Can you work these out from the drawing? Everything is in mm from the part's minimum corner. A direction names the side the tool comes from. Round coordinates to 2 decimals unless told otherwise and drop trailing zeros. One line per item, written item: value.
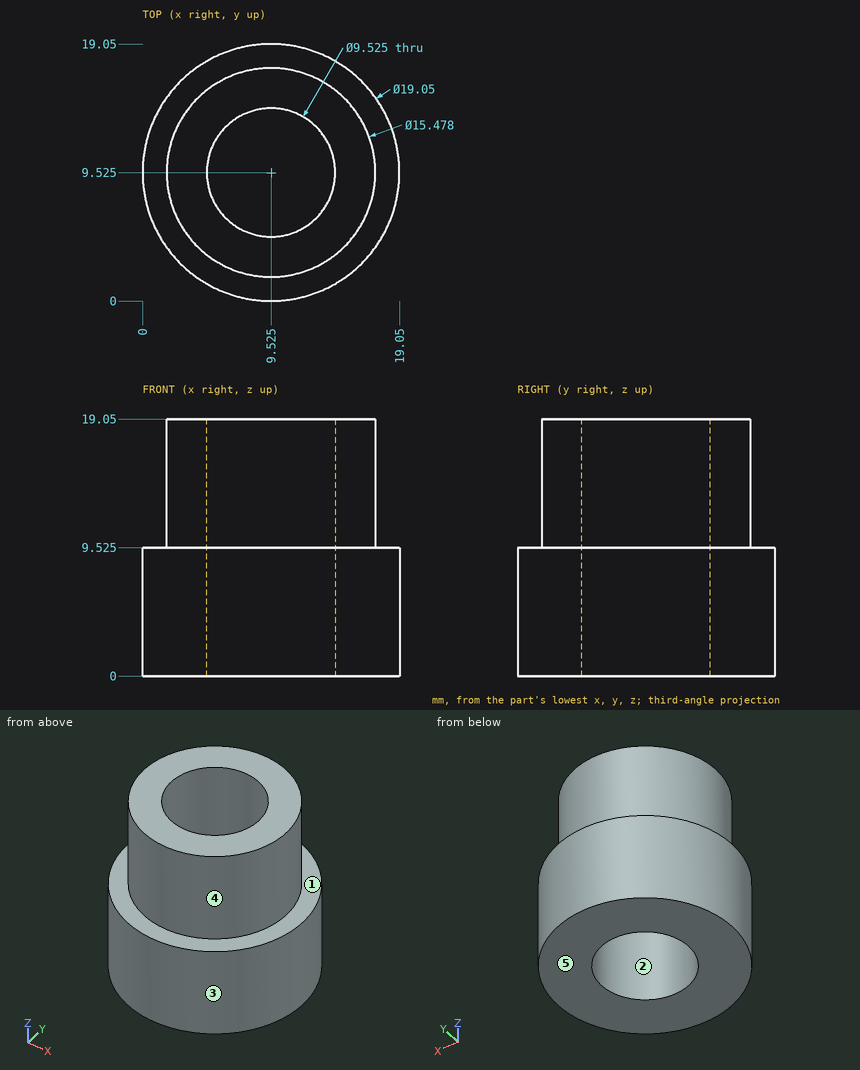
Item 1: For the marked faces 4 and 5, which set-ups out of +Z, -Z, +X, -X, +Y, -Y let a thin tool reach every point of the face, with its end or its side?
Output:
face 4: +Z
face 5: -Z, +X, -X, +Y, -Y
Item 2: If we mould it in two halves opening along X, with no side actions, what happens to the marked faces 1, 2 and 3? For each: released by +X, released by -X, zero draft, split by the parting line, or undercut.
Output:
face 1: zero draft
face 2: undercut
face 3: split by the parting line
Item 3: I need wall thicknesses on line 1 (X direction, y = 8.25, z = 12.75); line 2 (X direction, y = 11.25, z = 9); line 3 (Z direction, x = 16, y = 16.25) (3 decimals). Which ranges of each line are inside material? Lowest first, please. Write a range as from..to.
Output:
line 1: x = 1.89..4.94, 14.11..17.16
line 2: x = 0.16..5.09, 13.96..18.89
line 3: z = 0..9.525
Item 4: Will these pins go through, and if not, where does the flat tip stop? pin 1 Ø4 at (x, z) = (14, 10) entering from -Y; pin 2 Ø1 at (y, z) = (7, 3.5) entering from -X; pin 3 Ø1.5 at (x, z) = (11.5, 12) entering from +Y.
Output:
pin 1: stops at y = 0.34
pin 2: stops at x = 0.22
pin 3: stops at y = 17.17
